```python
from build123d import *

# Parameters (mm, degrees)
CUT_EXTRUDE_1_DEPTH = 3


with BuildPart() as part:
    # 草图1 → 旋转1 (revolve)
    with BuildSketch(Plane.XY, mode=Mode.PRIVATE) as revolve_1_sk:
        Polygon((0, 0), (0, 5), (4.5, 5), (4.5, 3), (69.5, 3), (69.5, 2.5), (79.25, 2.5), (79.25, 0), align=None)
    revolve(revolve_1_sk.sketch.rotate(Axis((0, 0, 0), (1, 0, 0)), 90), axis=Axis((0, 0, 0), (1, 0, 0)))

    # 草图2 → 切除-拉伸1 (cut)
    with BuildSketch(Plane.ZY):
        Polygon((0, 2.886751346), (-2.5, 1.443375673), (-2.5, -1.443375673), (0, -2.886751346), (2.5, -1.443375673), (2.5, 1.443375673), align=None)
    extrude(amount=-CUT_EXTRUDE_1_DEPTH, mode=Mode.SUBTRACT)


solid = part.part
```
Work out the finished part from the listing and answer in its coordinate system (mm). A direction names the side the tool comes from. Give positions to 0.01 mm unless a question says otherwise; leave off trailing zeros. Write each loop counter-clockwise with the first axis right and the second up, starting at its lowest first coordinate (ties: lowest second). Pieces come first, ordered by that corner, then holes.
(1) The part is cut by section C-C on x = 46. Write down the section's boundary in (y, z), plus the area to 3 significant figures.
Final values:
outline: circle Ø6 at (0, 0)
area: 28.3 mm2
(2) Which of the six approach directions +Z, -Z, +X, -X, +Y, -Y give full straight-line access (tool end or side, diameter ignored) to faces 1 (the cylindrical face through (2, 0, -5)), 2 (the flat face through (1.479, -2.155, -1.267)), 3 (the cylindrical face through (74.4, -0.1, -2.5))?
Final values:
face 1: +X, -X
face 2: -X
face 3: +X
(3) The mould has two halves that part along Z. Classify faces 4 (the flat face through (4.5, -0.1, 3.3)), 5 (the flat face through (1, 0, 2.5)), 6 (the cylindrical face through (37.46, -0.9, 2.86)): pulls with the +Z half, pulls with the -Z half, needs draft (parallel to the pull), parting line crosses it, or undercut.
Final values:
face 4: needs draft
face 5: undercut
face 6: parting line crosses it
(4) Straight lines are drawn through the part: line 1 (X direction, y = 0, z = -3.25); line 2 (Z direction, x = 38, y = 0.25); line 3 (X direction, y = 1.5, z = 1.75). For each, find the intervals that lie inside material, in ascending order.
Final values:
line 1: x = 0 to 4.5
line 2: z = -2.99 to 2.99
line 3: x = 3 to 79.25
(5) The part is cut by section A-A on y = 0. Write down the section's boundary in (x, z), plus the area to 3 significant figures.
Final values:
outline: (0, -5) - (4.5, -5) - (4.5, -3) - (69.5, -3) - (69.5, -2.5) - (79.25, -2.5) - (79.25, 2.5) - (69.5, 2.5) - (69.5, 3) - (4.5, 3) - (4.5, 5) - (0, 5) - (0, 2.5) - (3, 2.5) - (3, -2.5) - (0, -2.5) - close
area: 469 mm2
(6) The part is cut by section B-B on z = -1.75. Write down the section's boundary in (x, y).
Final values:
outline: (0, -4.68) - (4.5, -4.68) - (4.5, -2.44) - (69.5, -2.44) - (69.5, -1.79) - (79.25, -1.79) - (79.25, 1.79) - (69.5, 1.79) - (69.5, 2.44) - (4.5, 2.44) - (4.5, 4.68) - (0, 4.68) - (0, 1.88) - (3, 1.88) - (3, -1.88) - (0, -1.88) - close
(7) Flat-ended cylindrical pins translate along their axes: pin 1 Ø2 at (x, y) = (36.5, 0) entering from +Z; pin 2 Ø1.5 at (x, y) = (26.5, 1) entering from -Z; pin 3 Ø6 at (x, z) = (64, -0.5) entering from -Y. Find the tip coordinate at first contact, or state that the pin passes through.
Final values:
pin 1: stops at z = 3
pin 2: stops at z = -2.99
pin 3: stops at y = -3
